The listing builds one solid part. Answer for the finished solid, in the listing's coordinates (mm). A direction names the side the tool comes from. Coordinates: 2 decimals unless noted, no trailing zeros. Order: outer loops, then holes, each group sorted by start corner. A loop starts at its lowest first (then second) coordinate and runs counter-clockwise, first axis right, second up. Notation, with made-up numbers: (-2.5, 79.25) -> (3.5, 79.25) arc R11 cw to (3.5, 87.25) -> close; hole circle Ø8 at (10.25, 52). An arc over 180 degrees is marked (long way). Return JSON: item names as keys, results as strings.
```python
from build123d import *

# Parameters (mm, degrees)
SKETCH1_R                    = 50
BOSS_EXTRUDE1_DEPTH          = 40
FILLET1_R                    = 5
SKETCH2_R                    = 20
BOSS_EXTRUDE2_DEPTH          = 20
M33_TAPPED_HOLE1_D           = 29.5
M33_TAPPED_HOLE1_DEPTH       = 20
M33_TAPPED_HOLE1_CSINK_D     = 33.05
M33_TAPPED_HOLE1_CSINK_ANGLE = 90
M33_TAPPED_HOLE1_TIP         = 8.862694131
FILLET2_R                    = 5


with BuildPart() as part:
    # Sketch1 → Boss-Extrude1 (new, symmetric)
    with BuildSketch(Plane.XY):
        with BuildLine():
            Line((-60, 0), (-60, 80))
            Line((-60, 80), (60, 80))
            Line((60, 80), (60, 0))
            ThreePointArc((60, 0), (0, -60), (-60, 0))
        make_face()
        Circle(SKETCH1_R, mode=Mode.SUBTRACT)
    extrude(amount=BOSS_EXTRUDE1_DEPTH, both=True)

    # Fillet1
    fillet1_edges = [part.edges().sort_by_distance(p)[0] for p in [
        (-60, 80, 0),
        (60, 80, 0),
    ]]
    fillet(fillet1_edges, radius=FILLET1_R)

    # Sketch2 → Boss-Extrude2 (add)
    with BuildSketch(Plane(origin=(0, 80, 0), x_dir=(1, 0, 0), z_dir=(0, 1, 0))):
        with Locations(Location((0, 0, 0), (0, 0, 90))):
            Circle(SKETCH2_R)
    extrude(amount=BOSS_EXTRUDE2_DEPTH)

    # M33 Tapped Hole1
    with Locations(Plane.ZX.offset(100)):
        with Locations((0, 0)):
            CounterSinkHole(M33_TAPPED_HOLE1_D / 2, M33_TAPPED_HOLE1_CSINK_D / 2, depth=M33_TAPPED_HOLE1_DEPTH, counter_sink_angle=M33_TAPPED_HOLE1_CSINK_ANGLE)
            with Locations((0, 0, -(M33_TAPPED_HOLE1_DEPTH + M33_TAPPED_HOLE1_TIP / 2))):  # 118° drill point
                Cone(0, M33_TAPPED_HOLE1_D / 2, M33_TAPPED_HOLE1_TIP, mode=Mode.SUBTRACT)

    # Fillet2
    fillet2_edges = [part.edges().sort_by_distance(p)[0] for p in [
        (0, 80, 20),
    ]]
    fillet(fillet2_edges, radius=FILLET2_R)


solid = part.part
```
Item 1: The part is cut by section D-D on y = 77.5. Determine the outline of the cut face in (x, z).
Answer list:
{"outline": "(-59.33, -40) -> (59.33, -40) -> (59.33, 40) -> (-59.33, 40) -> close; hole circle Ø21.18 at (0, 0)"}
Item 2: The part is cut by section B-B on x = -42. Determine the outline of the cut face in (y, z).
Answer list:
{"outline": "(-42.85, -40) -> (-27.13, -40) -> (-27.13, 40) -> (-42.85, 40) -> close; (27.13, -40) -> (80, -40) -> (80, 40) -> (27.13, 40) -> close"}
Item 3: Flat-ended cylindrical pins translate along their axes: pin 1 (6 mm diameter, centred on x = 43.5, z = -26, fed in from +Y); pin 2 (6 mm diameter, centred on x = -18, z = -17, fed in from -Y); pin 3 (5 mm diameter, centred on x = 4, z = 16.5, fed in from -Y). Find the tip coordinate at first contact, or state that the pin passes through.
Answer list:
{"pin 1": "y = 80", "pin 2": "y = -58.09", "pin 3": "y = -59.98"}
Item 4: Find the intervals of material crossed by probe 1 along X at (y, z) = (85.25, 0); probe 2 along Y at (x, z) = (4, -30); probe 3 along Y at (x, z) = (-23, -34), in increasing order.
Answer list:
{"probe 1": "-20 to -14.75, 14.75 to 20", "probe 2": "-59.87 to -49.84, 49.84 to 80", "probe 3": "-55.42 to -44.4, 44.4 to 80"}
Item 5: Determine the mould class of faces 3 (the flat face through (1, 58, -40)), 4 (the cylindrical face through (-59, 78, -1)), 5 (the cylindrical face through (4.43, 88.98, -14.07)) for opening direction X: pulls with the +X half, pulls with the -X half, needs draft (parallel to the pull), parting line crosses it, or undercut.
Answer list:
{"face 3": "needs draft", "face 4": "pulls with the -X half", "face 5": "undercut"}
Item 6: The part is cut by section A-A on y = 23.5. Determine the outline of the cut face in (x, z).
Answer list:
{"outline": "(-60, -40) -> (-44.13, -40) -> (-44.13, 40) -> (-60, 40) -> close; (44.13, -40) -> (60, -40) -> (60, 40) -> (44.13, 40) -> close"}
Item 7: Which of the six approach directions +Z, -Z, +X, -X, +Y, -Y give full straight-line access (tool end or side, diameter ignored) to faces 1 (the cylindrical face through (1.319, -59.985, 0.56)), 2 (the cylindrical face through (19.524, 92.395, 4.336))?
Answer list:
{"face 1": "+Z, -Z, -Y", "face 2": "+Y"}
Item 8: The part is cut by section C-C on z = 32. Determine the outline of the cut face in (x, y), plus the area to 3 significant figures.
Answer list:
{"outline": "(-60, 0) arc R60 ccw to (60, 0) -> (60, 75) arc R5 ccw to (55, 80) -> (-55, 80) arc R5 ccw to (-60, 75) -> close; hole circle Ø100 at (0, 0)", "area": "7,390 mm2"}
